Geometry check sheet. Reference: the model listing, model coordinates, mm. Coordinates: 2 decimals unless noted, no trailing zeros. Loops run counter-clockwise (first coordinate to the right, second up) from the corner with the lowest first, then second, coordinate; pieces in that order, holes last.
from build123d import *

# Parameters (mm, degrees)
SKETCH015_R        = 51
SKETCH015_R_2      = 1.5
PAD013_DEPTH       = 3
POCKET_DEPTH       = 291.562952
POLARPATTERN_COUNT = 8


with BuildPart() as part:
    # Sketch015 → Pad013 (new body)
    with BuildSketch(Plane.XY):
        Circle(SKETCH015_R)
        with Locations((15.375, 26.630281)):
            Circle(SKETCH015_R_2, mode=Mode.SUBTRACT)
        with Locations((-30.75, 0)):
            Circle(SKETCH015_R_2, mode=Mode.SUBTRACT)
        with Locations((15.375, -26.630281)):
            Circle(SKETCH015_R_2, mode=Mode.SUBTRACT)
    extrude(amount=-PAD013_DEPTH)

    # Sketch017 (on Face6 of Pad013) → Pocket (cut, through all)
    with BuildSketch(Plane(origin=(0, 0, -3), x_dir=(1, 0, 0), z_dir=(0, 0, -1))):
        with BuildLine():
            ThreePointArc((8.022472, 46.919079), (0, 47.6), (-8.022472, 46.919079))
            ThreePointArc((-8.022472, 46.919079), (-10.555654, 43.340952), (-6.977528, 40.80777))
            ThreePointArc((6.977528, 40.80777), (0, 41.4), (-6.977528, 40.80777))
            ThreePointArc((6.977528, 40.80777), (10.555654, 43.340952), (8.022472, 46.919079))
        make_face()
    pocket = extrude(amount=-POCKET_DEPTH, mode=Mode.SUBTRACT)

    # PolarPattern: Pocket ×8 about axis
    polarpattern_axis = Axis((0, 0, -3), (0, 0, -1))
    for i in range(1, POLARPATTERN_COUNT):
        add(pocket.rotate(polarpattern_axis, i * 360 / POLARPATTERN_COUNT), mode=Mode.SUBTRACT)


solid = part.part
(1) Sectioned sample at B-B on y = 0. Record the cut outline in (x, z).
Findings:
outline: (-51, -3) - (-47.6, -3) - (-47.6, 0) - (-51, 0) - close; (-41.4, -3) - (-32.25, -3) - (-32.25, 0) - (-41.4, 0) - close; (-29.25, -3) - (41.4, -3) - (41.4, 0) - (-29.25, 0) - close; (47.6, -3) - (51, -3) - (51, 0) - (47.6, 0) - close
(2) Draft check along Y on faces 1 (the flat face through (-1, 1, -3)), 2 (the cylindrical face through (-10.543, 43.274, -1.521)). Enter one of: +Y half, -Y half, draft (parallel to the pull), parting line (faces both ways), or undercut.
Findings:
face 1: draft
face 2: undercut
(3) Gauge pin test, flat ends, axial feed: pin 1 Ø4 at (x, y) = (-30.75, 0) entering from -Z; pin 2 Ø1.5 at (y, z) = (-10.5, -0.5) entering from -X; pin 3 Ø1 at (y, z) = (18.5, -2) entering from -X. Record the tip position at first contact, or that the pin passes through.
Findings:
pin 1: stops at z = -3
pin 2: stops at x = -50.06
pin 3: stops at x = -47.72
(4) Sectioned sample at C-C on x = 44. Record the cut outline in (y, z), and give its area (3 significant figures).
Findings:
outline: (-25.79, -3) - (-10.6, -3) - (-10.6, 0) - (-25.79, 0) - close; (10.6, -3) - (25.79, -3) - (25.79, 0) - (10.6, 0) - close
area: 91.1 mm2
(5) Sectioned sample at D-D on y = -37. Record the cut outline in (x, z), and give its area (3 significant figures).
Findings:
outline: (-35.1, -3) - (-29.95, -3) - (-29.95, 0) - (-35.1, 0) - close; (-22.69, -3) - (22.69, -3) - (22.69, 0) - (-22.69, 0) - close; (29.95, -3) - (35.1, -3) - (35.1, 0) - (29.95, 0) - close
area: 167 mm2
(6) Sectioned sample at A-A on x = 0. Record the cut outline in (y, z), and give its area (3 significant figures).
Findings:
outline: (-51, -3) - (-47.6, -3) - (-47.6, 0) - (-51, 0) - close; (-41.4, -3) - (41.4, -3) - (41.4, 0) - (-41.4, 0) - close; (47.6, -3) - (51, -3) - (51, 0) - (47.6, 0) - close
area: 269 mm2
(7) Scan lines: L1, parallel to X at y = -35, z = -0.85; L2, parallel to X at y = -8, z = -2.05; L3, parallel to Y at x = 9, z = -0.25. Record each from-to range of solid material in increasing order.
Findings:
L1: x = -37.09 to -32.26, -22.91 to 22.91, 32.26 to 37.09
L2: x = -50.37 to -46.92, -40.8 to 40.8, 46.92 to 50.37
L3: y = -50.2 to -46.58, -41.15 to 41.15, 46.58 to 50.2
